from build123d import *

# Parameters (mm, degrees)
SKETCH1_R           = 1.35
BOSS_EXTRUDE1_DEPTH = 3
CHAMFER1_SIZE       = 3
SKETCH3_W           = 10
SKETCH3_H           = 15
SKETCH3_W_2         = 15
SKETCH3_W_3         = 8
BOSS_EXTRUDE2_DEPTH = 20
SKETCH4_R           = 1.25
CUT_EXTRUDE1_DEPTH  = 15
CHAMFER2_SIZE       = 1.5
CUT_EXTRUDE2_DEPTH  = 8
SKETCH2_R           = 9
CUT_EXTRUDE3_DEPTH  = 3
SKETCH6_R           = 3
BOSS_EXTRUDE3_DEPTH = 4
SKETCH7_R           = 0.9
CUT_EXTRUDE4_DEPTH  = 7
CHAMFER3_SIZE       = 2


with BuildPart() as part:
    # Sketch1 → Boss-Extrude1 (new body)
    with BuildSketch(Plane.XY):
        with BuildLine():
            Line((19, 44.2), (19, 38.2))
            Line((19, 38.2), (13, 38.2))
            ThreePointArc((13, 38.2), (6.5, 44.7), (0, 38.2))
            Line((0, 38.2), (0, 0))
            ThreePointArc((0, 0), (6.5, -6.5), (13, 0))
            Line((13, 0), (19, 0))
            Line((19, 0), (19, -6))
            Line((19, -6), (21, -8))
            Line((21, -8), (26, -8))
            Line((26, -8), (28, -6))
            Line((28, -6), (28, 0))
            Line((28, 0), (104, 0))
            Line((104, 0), (104, -6))
            Line((104, -6), (106, -8))
            Line((106, -8), (111, -8))
            Line((111, -8), (113, -6))
            Line((113, -6), (113, 0))
            Line((113, 0), (142.5, 0))
            Line((142.5, 0), (142.5, 38.2))
            Line((142.5, 38.2), (28, 38.2))
            Line((28, 38.2), (28, 44.114771772))
            Line((28, 44.114771772), (26, 46.2))
            Line((26, 46.2), (21, 46.2))
            Line((21, 46.2), (19, 44.2))
        make_face()
        with Locations((23.5, 42.2)):
            Circle(SKETCH1_R, mode=Mode.SUBTRACT)
        with Locations((108.5, 32)):
            Circle(SKETCH1_R, mode=Mode.SUBTRACT)
        with Locations((108.5, -4)):
            Circle(SKETCH1_R, mode=Mode.SUBTRACT)
        with Locations((23.5, -4)):
            Circle(SKETCH1_R, mode=Mode.SUBTRACT)
    extrude(amount=BOSS_EXTRUDE1_DEPTH)

    # Chamfer1
    chamfer1_edges = [part.edges().sort_by_distance(p)[0] for p in [
        (142.5, 19.1, 3),
    ]]
    chamfer(chamfer1_edges, length=CHAMFER1_SIZE - 0.0001)  # a hair under: the kernel refuses the full size

    # Sketch3 → Boss-Extrude2 (add)
    with BuildSketch(Plane.XY.offset(3)):
        with Locations((109, 17.9)):
            Rectangle(SKETCH3_W, SKETCH3_H)
        with Locations((56, 17.9)):
            Rectangle(SKETCH3_W_2, SKETCH3_H)
        with Locations((4, 17.9)):
            Rectangle(SKETCH3_W_3, SKETCH3_H)
    extrude(amount=BOSS_EXTRUDE2_DEPTH)

    # Sketch4 → Cut-Extrude1 (cut)
    with BuildSketch(Plane(origin=(0, 25.4, 0), x_dir=(1, 0, 0), z_dir=(0, 1, 0))):
        with Locations(Location((58.5, -18, 0), (0, 0, 180))):
            Circle(SKETCH4_R)
        with Locations(Location((53.5, -18, 0), (0, 0, 180))):
            Circle(SKETCH4_R)
        with Locations(Location((53.5, -8, 0), (0, 0, 180))):
            Circle(SKETCH4_R)
        with Locations(Location((58.5, -8, 0), (0, 0, 180))):
            Circle(SKETCH4_R)
        with Locations(Location((109, -18, 0), (0, 0, 180))):
            Circle(SKETCH4_R)
        with Locations(Location((3, -18, 0), (0, 0, 180))):
            Circle(SKETCH4_R)
        with Locations(Location((3, -8, 0), (0, 0, 180))):
            Circle(SKETCH4_R)
        with Locations(Location((109, -8, 0), (0, 0, 180))):
            Circle(SKETCH4_R)
    extrude(amount=-CUT_EXTRUDE1_DEPTH, mode=Mode.SUBTRACT)

    # Chamfer2
    chamfer2_edges = [part.edges().sort_by_distance(p)[0] for p in [
        (114, 10.4, 13),
        (114, 25.4, 13),
        (104, 25.4, 13),
        (104, 10.4, 13),
        (63.5, 10.4, 13),
        (63.5, 25.4, 13),
        (48.5, 25.4, 13),
        (48.5, 10.4, 13),
        (8, 10.4, 13),
        (8, 25.4, 13),
        (0, 25.4, 13),
        (0, 10.4, 13),
    ]]
    chamfer(chamfer2_edges, length=CHAMFER2_SIZE)

    # Sketch5 → Cut-Extrude2 (cut)
    with BuildSketch(Plane(origin=(0, 25.4, 0), x_dir=(1, 0, 0), z_dir=(0, 1, 0))):
        Polygon((3, -5.517393842), (0.85, -6.758696921), (0.85, -9.241303079), (3, -10.482606158), (5.15, -9.241303079), (5.15, -6.758696921), align=None)
        Polygon((3, -15.517393842), (0.85, -16.758696921), (0.85, -19.241303079), (3, -20.482606158), (5.15, -19.241303079), (5.15, -16.758696921), align=None)
        Polygon((53.5, -5.517393842), (51.35, -6.758696921), (51.35, -9.241303079), (53.5, -10.482606158), (55.65, -9.241303079), (55.65, -6.758696921), align=None)
        Polygon((58.5, -5.517393842), (56.35, -6.758696921), (56.35, -9.241303079), (58.5, -10.482606158), (60.65, -9.241303079), (60.65, -6.758696921), align=None)
        Polygon((58.5, -15.517393842), (56.35, -16.758696921), (56.35, -19.241303079), (58.5, -20.482606158), (60.65, -19.241303079), (60.65, -16.758696921), align=None)
        Polygon((53.5, -15.517393842), (51.35, -16.758696921), (51.35, -19.241303079), (53.5, -20.482606158), (55.65, -19.241303079), (55.65, -16.758696921), align=None)
        Polygon((109, -15.517393842), (106.85, -16.758696921), (106.85, -19.241303079), (109, -20.482606158), (111.15, -19.241303079), (111.15, -16.758696921), align=None)
        Polygon((109, -5.517393842), (106.85, -6.758696921), (106.85, -9.241303079), (109, -10.482606158), (111.15, -9.241303079), (111.15, -6.758696921), align=None)
    extrude(amount=-CUT_EXTRUDE2_DEPTH, mode=Mode.SUBTRACT)

    # Sketch2 → Cut-Extrude3 (cut)
    with BuildSketch(Plane(origin=(0, 0, 0), x_dir=(-1, 0, 0), z_dir=(0, 0, -1))):
        with Locations((-18, 19.1)):
            Circle(SKETCH2_R)
        with Locations((-85.5, 19.1)):
            Circle(SKETCH2_R)
        with Locations((-130.5, 19.1)):
            Circle(SKETCH2_R)
    extrude(amount=-CUT_EXTRUDE3_DEPTH, mode=Mode.SUBTRACT)

    # Sketch6 → Boss-Extrude3 (add)
    with BuildSketch(Plane.XY.offset(3)):
        with Locations((119, 33.1)):
            Circle(SKETCH6_R)
        with Locations((135, 33.1)):
            Circle(SKETCH6_R)
        with Locations(Location((135, 5.1, 0), (0, 0, 180))):
            Circle(SKETCH6_R)
        with Locations(Location((119, 5.1, 0), (0, 0, 180))):
            Circle(SKETCH6_R)
    extrude(amount=BOSS_EXTRUDE3_DEPTH)

    # Sketch7 → Cut-Extrude4 (cut)
    with BuildSketch(Plane.XY.offset(7)):
        with Locations((135, 33.1)):
            Circle(SKETCH7_R)
        with Locations((119, 33.1)):
            Circle(SKETCH7_R)
        with Locations((119, 5.1)):
            Circle(SKETCH7_R)
        with Locations((135, 5.1)):
            Circle(SKETCH7_R)
    extrude(amount=-CUT_EXTRUDE4_DEPTH, mode=Mode.SUBTRACT)

    # Chamfer3
    chamfer3_edges = [part.edges().sort_by_distance(p)[0] for p in [
        (56, 25.4, 3),
        (4, 25.4, 3),
        (109, 25.4, 3),
    ]]
    chamfer(chamfer3_edges, length=CHAMFER3_SIZE)


solid = part.part
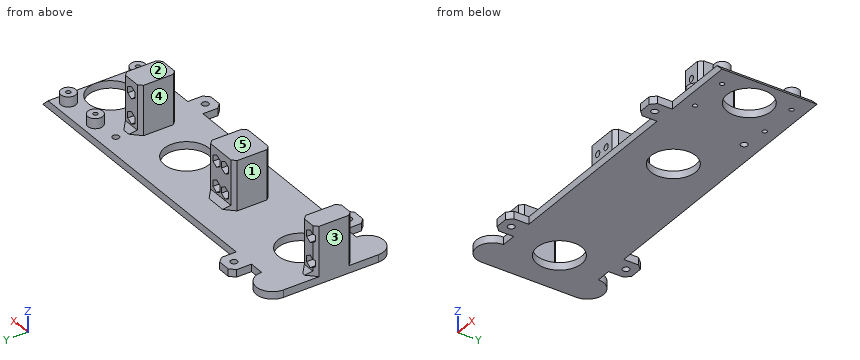
Could you check a few things on this model? Use its own coordinates, in mm. Face numbers are marked on the shaded views. A direction names the side the tool comes from. Round coordinates to 2 decimals unless told otherwise and drop trailing zeros. Write each loop counter-clockwise with the first axis right and the second up, starting at its lowest first coordinate (ties: lowest second). Pieces come first, ordered by that corner, then holes. Notation, with made-up numbers: (23.25, 26.5) - (70.25, 26.5) arc R21 cw to (70.25, 50.5) - close; hole circle Ø7 at (-13, 57). An arc over 180 degrees is marked (long way). Put each result on its own line as item: value. Start each with the question number.
(1) I want a section at B-B, the plane x = 102.5. Please give me the cut outline in (y, z), plus the area to 3 significant figures.
(2) Will these pins go through, and if not, where does the flat tip stop? pin 1 (2 mm diameter, centred on x = 79.5, y = 8, fed in from +Z); pin 2 (4 mm diameter, centred on x = 62, z = 3, fed in from -Y); pin 3 (0.9 mm diameter, centred on x = 75.5, z = 2, fed in from +Y).
(3) Thinking about a two-plate mould opening in X: for the marked faces 1, 2 and 3, which applies, released by +X, released by -X, zero draft, split by the parting line, or undercut?
(4) I want a section at A-A, the plane x = 85.5. Please give me the cut outline in (y, z).
(5) For the marked faces 4 and 5, which set-ups out of +Z, -Z, +X, -X, +Y, -Y let a thin tool reach every point of the face, with its end or its side?
(6) I need wall thicknesses on probe 1 along Y at (x, z) = (108.5, 0.6); probe 2 along Y at (x, z) = (119, 4); probe 3 along Z at (x, y) = (3, 13.25). Which ranges of each line are inside material? Lowest first, please.
Here are the results:
1. outline: (0, 0) - (38.2, 0) - (38.2, 3) - (0, 3) - close
1. area: 115 mm^2
2. pin 1: stops at z = 3
2. pin 2: stops at y = 0
2. pin 3: stops at y = 38.2
3. face 1: undercut
3. face 2: zero draft
3. face 3: released by -X
4. outline: (0, 0) - (10.1, 0) - (10.1, 3) - (0, 3) - close; (28.1, 0) - (38.2, 0) - (38.2, 3) - (28.1, 3) - close
5. face 4: +Z, +Y, -Y
5. face 5: +Z, +X, -X, +Y, -Y
6. probe 1: y = -8 to -5.35, -2.65 to 30.65, 33.35 to 38.2
6. probe 2: y = 2.1 to 4.2, 6 to 8.1, 30.1 to 32.2, 34 to 36.1
6. probe 3: z = 0 to 6.75, 9.25 to 16.75, 19.25 to 23
